Part model, mm, in its own coordinate system. A direction names the side the tool comes from. Give positions to 0.01 mm unless a question says otherwise; leave off trailing zeros. Loops run counter-clockwise (first coordinate to the right, second up) from the corner with the lowest first, then second, coordinate; pieces in that order, holes last. Notation, with made-up numbers: (57.25, 49) -> (61.25, 49) arc R29 cw to (61.25, 79) -> close; hole circle Ø3 at (52.25, 61). An arc over 180 degrees is marked (long way). One line per question, with ' | ' between items.
```python
from build123d import *

# Parameters (mm, degrees)
SKETCH6_R               = 19.175
SKETCH6_R_2             = 16
BOSS_EXTRUDE4_DEPTH     = 5
BOSS_EXTRUDE6_REACH     = 11.175
SKETCH8_W               = 15
SKETCH8_H               = 10
SKETCH7_2_R             = 4
CUT_EXTRUDE1_DEPTH      = 16.475
CUT_EXTRUDE1_DEPTH_BACK = 23.875


with BuildPart() as part:
    # Sketch6 → Boss-Extrude4 (new body, symmetric)
    with BuildSketch(Plane(origin=(0, 0, 0), x_dir=(1, 0, 0), z_dir=(0, 1, 0))):
        Circle(SKETCH6_R)
        Circle(SKETCH6_R_2, mode=Mode.SUBTRACT)
    extrude(amount=BOSS_EXTRUDE4_DEPTH, both=True)

    # Sketch8 → Boss-Extrude6 (add, up to next)
    with BuildSketch(Plane.XY.offset(-10), mode=Mode.PRIVATE) as boss_extrude6_sk1:
        Rectangle(SKETCH8_W, SKETCH8_H)
    boss_extrude6_tool1 = extrude(boss_extrude6_sk1.sketch, amount=-BOSS_EXTRUDE6_REACH, mode=Mode.PRIVATE) - part.part
    add(boss_extrude6_tool1.solids().sort_by_distance((0, 0, -10))[0])

    # Sketch7<2> → Cut-Extrude1 (cut, two sides)
    with BuildSketch(Plane.XY.offset(3.7)) as cut_extrude1_sk:
        Circle(SKETCH7_2_R)
    extrude(amount=CUT_EXTRUDE1_DEPTH, mode=Mode.SUBTRACT)
    extrude(cut_extrude1_sk.sketch, amount=-CUT_EXTRUDE1_DEPTH_BACK, mode=Mode.SUBTRACT)


solid = part.part
```
1) Tool access for faces 4 (the flat face through (0, 5, -11)), 5 (the flat face through (-0.1, -4.4, -10)): list every direction of +Z, -Z, +X, -X, +Y, -Y with a clear straight run to the whole face (end or side of a thin tool).
Found:
face 4: +Z, -Z, +X, -X, +Y | face 5: +Y, -Y
2) Drill centre lines: line 1 (Y direction, x = 0, z = -12.5); line 2 (X direction, y = 0.75, z = -12.5); line 3 (X direction, y = -0.5, z = 0) (3 decimals). Where is each one in solid material? Low to high.
Found:
line 1: -5 to -4, 4 to 5 | line 2: -14.54 to -9.99, -7.5 to -3.93, 3.93 to 7.5, 9.99 to 14.54 | line 3: -19.175 to -16, 16 to 19.175
3) Saw through at D-D (x = 0). Give the cut face in (y, z) (3 decimals).
Found:
outline: (-5, -19.175) -> (-4, -19.175) -> (-4, -10) -> (-5, -10) -> close; (-5, 16) -> (-4, 16) -> (-4, 19.175) -> (-5, 19.175) -> close; (4, -19.175) -> (5, -19.175) -> (5, -10) -> (4, -10) -> close; (4, 16) -> (5, 16) -> (5, 19.175) -> (4, 19.175) -> close
4) Saw through at C-C (x = -15.5). Give the cut face in (y, z), and give its area (3 significant figures).
Found:
outline: (-5, -11.29) -> (5, -11.29) -> (5, -3.97) -> (-5, -3.97) -> close; (-5, 3.97) -> (5, 3.97) -> (5, 11.29) -> (-5, 11.29) -> close | area: 146 mm2
5) Pull direction Z, two halves, no side cores. Call faces 1 (the cylindrical face through (8.85, 0.07, 17.01)), 2 (the cylindrical face through (-0.867, -3.905, -14.523)), 3 (the flat face through (7.5, 0, -12)): pulls with the +Z half, pulls with the -Z half, needs draft (parallel to the pull), parting line crosses it, or undercut.
Found:
face 1: parting line crosses it | face 2: needs draft | face 3: undercut
6) Saw through at A-A (z = 0). Give the cut face in (x, y) (3 decimals), and give its area (3 significant figures).
Found:
outline: (-19.175, -5) -> (-16, -5) -> (-16, 5) -> (-19.175, 5) -> close; (16, -5) -> (19.175, -5) -> (19.175, 5) -> (16, 5) -> close | area: 63.5 mm2
7) Pin check, flat tips, straight feed: P1, Ø1.2, axis at y = -1, z = -12, coming from the +X side; P2, Ø3.5, axis at y = -1.5, z = -12, coming from the -X side; P3, Ø3, axis at x = -15, y = -1.5, coming from the -Z side; P4, Ø3, axis at x = 4, z = -7.5, coming from the +Y side. Stop position of each tip, or through.
Found:
P1: x = 15.42 | P2: x = -16.21 | P3: z = -13.62 | P4: through
8) Saw through at B-B (y = 1). Give the cut face in (x, z) (3 decimals), and give its area (3 significant figures).
Found:
outline: (-7.5, -14.133) arc R16 cw to (-3.873, 15.524) -> (-3.873, 18.78) arc R19.175 ccw to (-3.873, -18.78) -> (-3.873, -10) -> (-7.5, -10) -> close; (3.873, -18.78) arc R19.175 ccw to (3.873, 18.78) -> (3.873, 15.524) arc R16 cw to (7.5, -14.133) -> (7.5, -10) -> (3.873, -10) -> close | area: 337 mm2
